Geometry check sheet. Reference: the model listing, model coordinates, mm. A direction names the side the tool comes from. Give positions to 0.01 mm unless a question says otherwise; leave off trailing zeros. Order: outer loops, then holes, each group sorted by start corner. A loop starts at its lowest first (then second) coordinate and runs counter-clockwise, first axis right, second up. Notation, with made-up numbers: M 80,11 L 138,11 A22 cw 138,39 Z; hole C 62,31.25 d8. An arc over 180 degrees is marked long. Answer as CSV lines item,"result". Start each with the question number.
Q1. Set-up check for faces 4 (the cylindrical face through (-24.94, -0.54, 2.44)), 5 (the cylindrical face through (0.29, 4.77, -1.5)), 6 (the flat face through (21, 2, 2)): record each of +Z, -Z, +X, -X, +Y, -Y from which the full face is reachable in a straight line by a thin tool's end or side.
Q2. Go/stop test with flat-tipped pins: pin 1 (1 mm diameter, centred on x = -16, y = -4, fed in from -Z); pin 2 (1.5 mm diameter, centred on x = -15.5, y = -1, fed in from -Z). Record where each tip stops, or that it passes through.
Q3. Mould release check, pull along X, two halves, no side actions. Record for faces 1 (the cylindrical face through (0, -2, 0)), 2 (the flat face through (-21, -2, 2)), 3 (the cylindrical face through (25.06, -0.54, 2.44)): +X half, -X half, draft (parallel to the pull), parting line (faces both ways), or undercut.
Q4. Section check A-A, the plane y = 0. Record the boundary of the cut face in (x, z).
Q5. Section check C-C, the plane x = 0. Record the boundary of the cut face in (y, z).
Q6. Thickness scan on line 1 (X direction, y = 0, z = 1.75); line 2 (X direction, y = 0, z = -3.5); line 3 (Y direction, x = 0, z = 0.5). Record the ranges inside material, lowest first.
Q7. Section check D-D, the plane x = 14. Record the boundary of the cut face in (y, z), then the cut area to 3 significant figures.
Q8. Section check B-B, the plane z = 0. Record the boundary of the cut face in (x, y), then the cut area to 3 significant figures.
```python
from build123d import *

# Parameters (mm, degrees)
SKETCH_3_R          = 2
CUT_EXTRUDE_1_DEPTH = 10


with BuildPart() as part:
    # 草圖1 → 旋轉1 (revolve)
    with BuildSketch(Plane.XY):
        Polygon((-29, 0), (-29, 2.5), (-21, 2.5), (-21, 5), (21, 5), (21, 2.5), (29, 2.5), (29, 0), align=None)
    revolve(axis=Axis((29, 0, 0), (-1, 0, 0)))

    # 草圖3 → 除料-伸長1 (cut, symmetric)
    with BuildSketch(Plane.XY):
        Circle(SKETCH_3_R)
    extrude(amount=CUT_EXTRUDE_1_DEPTH, both=True, mode=Mode.SUBTRACT)


solid = part.part
```
Answer block:
1,face 4,"-X"
1,face 5,"+X, -X"
1,face 6,"+X"
2,pin 1,"stops at z = -3.57"
2,pin 2,"stops at z = -4.99"
3,face 1,"undercut"
3,face 2,"-X half"
3,face 3,"draft"
4,outline,"M -29,-2.5 L -21,-2.5 L -21,-5 L -2,-5 L -2,5 L -21,5 L -21,2.5 L -29,2.5 Z; M 2,-5 L 21,-5 L 21,-2.5 L 29,-2.5 L 29,2.5 L 21,2.5 L 21,5 L 2,5 Z"
5,outline,"M -2,-4.58 L -2,4.58 A5 ccw Z; M 2,-4.58 A5 ccw 2,4.58 Z"
6,line 1,"x = -29 to -2, 2 to 29"
6,line 2,"x = -21 to -2, 2 to 21"
6,line 3,"y = -4.97 to -2, 2 to 4.97"
7,outline,"C 0,0 d10"
7,area,"78.5 mm2"
8,outline,"M -29,-2.5 L -21,-2.5 L -21,-5 L 21,-5 L 21,-2.5 L 29,-2.5 L 29,2.5 L 21,2.5 L 21,5 L -21,5 L -21,2.5 L -29,2.5 Z; hole C 0,0 d4"
8,area,"487 mm2"
